from build123d import *

# Parameters (mm, degrees)
SKETCH1_R           = 18.5
SKETCH1_R_2         = 12.5
BOSS_EXTRUDE1_DEPTH = 7
CHAMFER1_SIZE       = 0.4


with BuildPart() as part:
    # Sketch1 → Boss-Extrude1 (new body)
    with BuildSketch(Plane(origin=(0, 0, 0), x_dir=(1, 0, 0), z_dir=(0, 1, 0))):
        with Locations(Location((0, 0, 0), (0, 0, 270))):
            Circle(SKETCH1_R)
        with Locations(Location((0, 0, 0), (0, 0, 270))):
            Circle(SKETCH1_R_2, mode=Mode.SUBTRACT)
    extrude(amount=BOSS_EXTRUDE1_DEPTH)

    # Chamfer1
    chamfer1_edges = [part.edges().sort_by_distance(p)[0] for p in [
        (0, 0, -18.5),
        (0, 7, -18.5),
        (0, 0, -12.5),
        (0, 7, -12.5),
    ]]
    chamfer(chamfer1_edges, length=CHAMFER1_SIZE)


solid = part.part
Design review of the part built by this model. Coordinates are the model's own, in mm. Coordinates: 2 decimals unless noted, no trailing zeros. Loops run counter-clockwise (first coordinate to the right, second up) from the corner with the lowest first, then second, coordinate; pieces in that order, holes last. Notation, with made-up numbers: (66.25, 27.25) -> (115.25, 27.25) arc R27 cw to (115.25, 45.25) -> close; hole circle Ø9 at (57, 79.25). An arc over 180 degrees is marked (long way). Use a Markdown table: item, result. Add a question column.
Item 1: We need section B-B, the plane x = 0. Write out the cut boundary in (y, z), and give its area (3 significant figures).
Item 2: We need section A-A, the plane z = 0. Write out the cut boundary in (x, y), and give its area (3 significant figures).
Item 3: Clearance check with flat-ended pins moving along their axes: P1, Ø1.5, axis at x = 1, y = 4, coming from the +Z side; P2, Ø1.5, axis at x = -7.5, y = 5.5, coming from the +Z side; P3, Ø2, axis at y = 2.5, z = 14.5, coming from the -X side. State where each tip first meets the part, or that it passes through.
Item 4: Wall thickness on L1, parallel to X at y = 4, z = 0; L2, parallel to X at y = 0.75, z = -3.5; L3, parallel to Z at x = 10, y = 6.5: over which ranges is each line inside the solid? List them lowest first. Write a range as from..to.
Item 5: We need section C-C, the plane y = 2.5. Write out the cut boundary in (x, z), and give its area (3 significant figures).
Item 6: The part is to be moulded in two halves that separate along Z. For faces 1 (the cylindrical face through (-7.086, 3.457, 17.089)), 2 (the flat face through (-12, 7, 8)), 3 (the cylindrical face through (3.755, 3.457, 11.923)), say which applies: +Z half, -Z half, draft (parallel to the pull), parting line (faces both ways), or undercut.
Numbers:
| question | item | result |
|---|---|---|
| 1 | outline | (0, -18.1) -> (0.4, -18.5) -> (6.6, -18.5) -> (7, -18.1) -> (7, -12.9) -> (6.6, -12.5) -> (0.4, -12.5) -> (0, -12.9) -> close; (0, 12.9) -> (0.4, 12.5) -> (6.6, 12.5) -> (7, 12.9) -> (7, 18.1) -> (6.6, 18.5) -> (0.4, 18.5) -> (0, 18.1) -> close |
| 1 | area | 83.4 mm^2 |
| 2 | outline | (-18.5, 0.4) -> (-18.1, 0) -> (-12.9, 0) -> (-12.5, 0.4) -> (-12.5, 6.6) -> (-12.9, 7) -> (-18.1, 7) -> (-18.5, 6.6) -> close; (12.5, 0.4) -> (12.9, 0) -> (18.1, 0) -> (18.5, 0.4) -> (18.5, 6.6) -> (18.1, 7) -> (12.9, 7) -> (12.5, 6.6) -> close |
| 2 | area | 83.4 mm^2 |
| 3 | P1 | stops at z = 18.5 |
| 3 | P2 | stops at z = 17.22 |
| 3 | P3 | stops at x = -12.65 |
| 4 | L1 | x = -18.5..-12.5, 12.5..18.5 |
| 4 | L2 | x = -18.17..-12, 12..18.17 |
| 4 | L3 | z = -15.56..-7.5, 7.5..15.56 |
| 5 | outline | circle Ø37 at (0, 0); hole circle Ø25 at (0, 0) |
| 5 | area | 584 mm^2 |
| 6 | face 1 | parting line |
| 6 | face 2 | draft |
| 6 | face 3 | undercut |
